Here's how the part is built. I have some questions about the finished solid (model axes, mm). Face numbers are marked on the shaded views. A direction names the side the tool comes from. Round coordinates to 2 decimals unless told otherwise and drop trailing zeros. Loops run counter-clockwise (first coordinate to the right, second up) from the corner with the lowest first, then second, coordinate; pieces in that order, holes last. Notation, with made-up numbers: M 85,12.5 L 118,12.5 A22 cw 118,28.5 Z; hole C -29.5,41.25 d2. An arc over 180 degrees is marked long. Use a Markdown table: item, result.
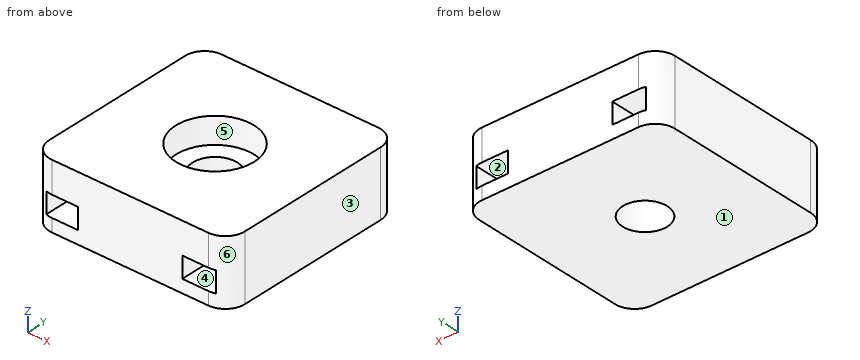
from build123d import *

# Parameters (mm, degrees)
BASE_15X15_DEPTH     = 5
CROQUIS2_R           = 1.7
PASO_M3_DEPTH        = 5
CAJA_CABEZA_START    = 3
CROQUIS3_R           = 3
CAJA_CABEZA_DEPTH    = 2
TUNEL_CINCHO_A_START = 4
CROQUIS4_W           = 1.6
CROQUIS4_H           = 16
TUNEL_CINCHO_A_DEPTH = 2.5
TUNEL_CINCHO_B_START = -6.5
CROQUIS5_W           = 1.6
CROQUIS5_H           = 16
TUNEL_CINCHO_B_DEPTH = 2.5


with BuildPart() as part:
    # Croquis1 → Base_15x15 (new body)
    with BuildSketch(Plane.XY):
        with BuildLine():
            Line((-6, -7.5), (6, -7.5))
            ThreePointArc((6, -7.5), (7.060660172, -7.060660172), (7.5, -6))
            Line((7.5, -6), (7.5, 6))
            ThreePointArc((7.5, 6), (7.060660172, 7.060660172), (6, 7.5))
            Line((6, 7.5), (-6, 7.5))
            ThreePointArc((-6, 7.5), (-7.060660172, 7.060660172), (-7.5, 6))
            Line((-7.5, 6), (-7.5, -6))
            ThreePointArc((-7.5, -6), (-7.060660172, -7.060660172), (-6, -7.5))
        make_face()
    extrude(amount=BASE_15X15_DEPTH)

    # Croquis2 → Paso_M3 (cut)
    with BuildSketch(Plane.XY):
        Circle(CROQUIS2_R)
    extrude(amount=PASO_M3_DEPTH, mode=Mode.SUBTRACT)

    # Croquis3 → Caja_cabeza (cut)
    with BuildSketch(Plane.XY.offset(CAJA_CABEZA_START)):
        Circle(CROQUIS3_R)
    extrude(amount=CAJA_CABEZA_DEPTH, mode=Mode.SUBTRACT)

    # Croquis4 → Tunel_cincho_A (cut)
    with BuildSketch(Plane(origin=(0, 0, 0), x_dir=(0, 0, -1), z_dir=(1, 0, 0)).offset(TUNEL_CINCHO_A_START)):
        with Locations((-1.8, 0)):
            Rectangle(CROQUIS4_W, CROQUIS4_H)
    extrude(amount=TUNEL_CINCHO_A_DEPTH, mode=Mode.SUBTRACT)

    # Croquis5 → Tunel_cincho_B (cut)
    with BuildSketch(Plane(origin=(0, 0, 0), x_dir=(0, 0, -1), z_dir=(1, 0, 0)).offset(TUNEL_CINCHO_B_START)):
        with Locations((-1.8, 0)):
            Rectangle(CROQUIS5_W, CROQUIS5_H)
    extrude(amount=TUNEL_CINCHO_B_DEPTH, mode=Mode.SUBTRACT)


solid = part.part
1. I need wall thicknesses on probe 1 along X at (y, z) = (0, 1.65); probe 2 along X at (y, z) = (1.25, 2.25); probe 3 along X at (y, z) = (3.75, 2.05). Which ranges of each line are inside material? Lowest first, please. Write a range as from..to.
Answer sheet:
| item | result |
|---|---|
| probe 1 | -7.5..-6.5, -4..-1.7, 1.7..4, 6.5..7.5 |
| probe 2 | -7.5..-6.5, -4..-1.15, 1.15..4, 6.5..7.5 |
| probe 3 | -7.5..-6.5, -4..4, 6.5..7.5 |
2. Imagine slicing it at D-D, the plane y = -4.5. Write out the boundary of the cut face in (x, z).
Answer sheet:
| item | result |
|---|---|
| outline | M -7.5,0 L 7.5,0 L 7.5,5 L -7.5,5 Z; hole M -6.5,1 L -4,1 L -4,2.6 L -6.5,2.6 Z; hole M 4,1 L 6.5,1 L 6.5,2.6 L 4,2.6 Z |
3. We'd pull the mould along Z, two halves only. Please class the marked faces 1, 2 and 3: +Z half, -Z half, draft (parallel to the pull), parting line (faces both ways), or undercut.
Answer sheet:
| item | result |
|---|---|
| face 1 | -Z half |
| face 2 | undercut |
| face 3 | draft |
4. Imagine slicing it at B-B, the plane y = 0. Write out the boundary of the cut face in (x, z), then the cut area to 3 significant figures.
Answer sheet:
| item | result |
|---|---|
| outline | M -7.5,0 L -1.7,0 L -1.7,3 L -3,3 L -3,5 L -7.5,5 Z; M 1.7,0 L 7.5,0 L 7.5,5 L 3,5 L 3,3 L 1.7,3 Z; hole M -6.5,1 L -4,1 L -4,2.6 L -6.5,2.6 Z; hole M 4,1 L 6.5,1 L 6.5,2.6 L 4,2.6 Z |
| area | 44.8 mm2 |
5. Which directions (+Z, -Z, +X, -X, +Y, -Y) give clear straight access to the entire face, cutting with the end or side of a thin tool? Please do the marked faces 4, 5 and 6.
Answer sheet:
| item | result |
|---|---|
| face 4 | +Y, -Y |
| face 5 | +Z |
| face 6 | +Z, -Z, +X, -Y |
6. Imagine slicing it at C-C, the plane z = 0.65. Write out the boundary of the cut face in (x, y), then the cut area to 3 significant figures.
Answer sheet:
| item | result |
|---|---|
| outline | M -7.5,-6 A1.5 ccw -6,-7.5 L 6,-7.5 A1.5 ccw 7.5,-6 L 7.5,6 A1.5 ccw 6,7.5 L -6,7.5 A1.5 ccw -7.5,6 Z; hole C 0,0 d3.4 |
| area | 214 mm2 |
7. Imagine slicing it at A-A, the plane x = 0. Write out the boundary of the cut face in (y, z), then the cut area to 3 significant figures.
Answer sheet:
| item | result |
|---|---|
| outline | M -7.5,0 L -1.7,0 L -1.7,3 L -3,3 L -3,5 L -7.5,5 Z; M 1.7,0 L 7.5,0 L 7.5,5 L 3,5 L 3,3 L 1.7,3 Z |
| area | 52.8 mm2 |
